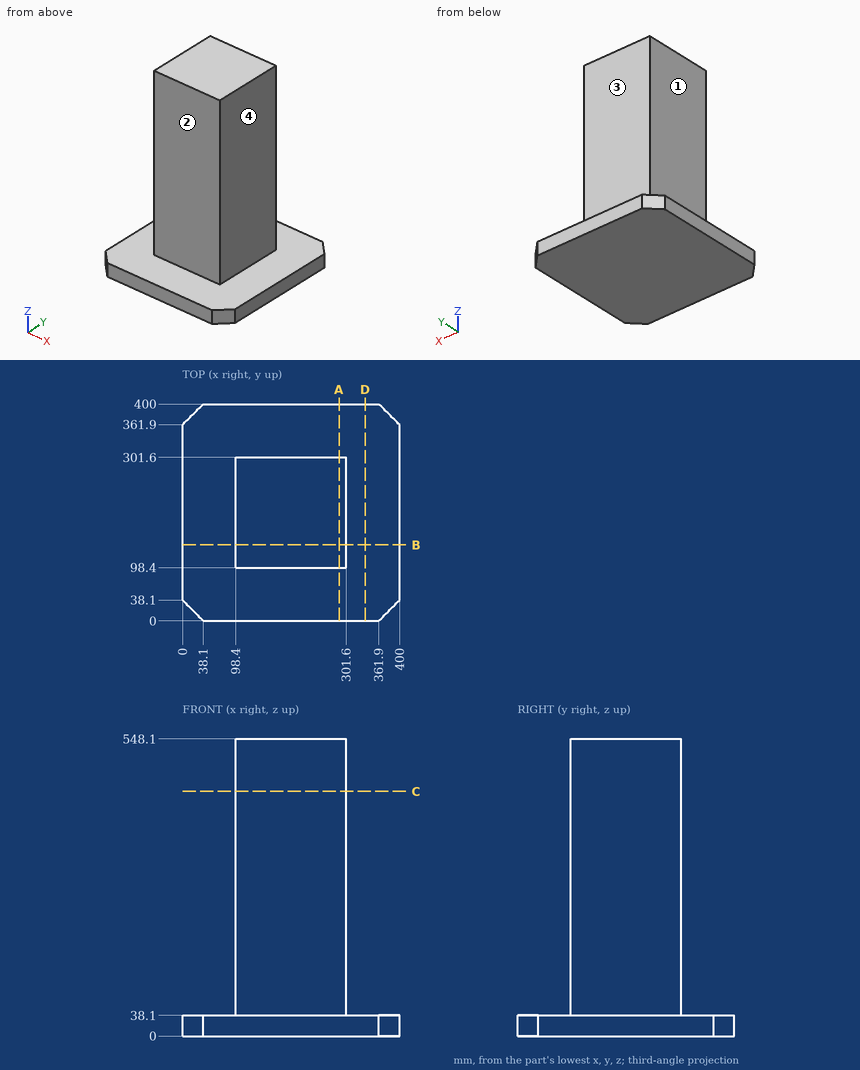
The drawing under review shows one solid part. Ordinate dimensions are in mm from its lowest x, y, z. A direction names the side the tool comes from. Give positions to 0.01 mm unless a question says otherwise; leave off trailing zeros. Write each loop counter-clockwise with the first axis right and the second up, starting at its lowest first coordinate (ties: lowest second). Pieces come first, ordered by that corner, then holes. Notation, with made-up numbers: (56, 33) -> (81, 33) arc R21 ccw to (81, 61) -> close; hole circle Ø9 at (-5.5, -10.5). An arc over 180 degrees is marked (long way). Use CSV: the item, a comma, the result in double quotes.
Q1. For P1, Ø1, axis at x = 122.5, z = 311.5, coming from the -Y side; P2, Ø1.5, axis at x = 269.5, y = 337, coming from the +Z side; P3, Ø4, axis at y = 180.5, z = 312.5, coming from the +X side, all flat-tipped, find the tip position at first contact; note any pin that passes through.
Conclusion:
P1,"y = 98.4"
P2,"z = 38.1"
P3,"x = 301.6"
Q2. Take a section at D-D, the plane x = 336.5. Write out the cut boundary in (y, z).
Conclusion:
outline,"(0, 0) -> (400, 0) -> (400, 38.1) -> (0, 38.1) -> close"
Q3. Take a section at C-C, the plane z = 451. Write out the cut boundary in (x, y).
Conclusion:
outline,"(98.4, 98.4) -> (301.6, 98.4) -> (301.6, 301.6) -> (98.4, 301.6) -> close"
Q4. To check wall thickness, follow probe 1 along X at (y, z) = (203.5, 42); probe 2 along Z at (x, y) = (313.5, 200.5). State the ranges of each line that lie inside material, in increasing order. Write a range as [from, to].
Conclusion:
probe 1,"[98.4, 301.6]"
probe 2,"[0, 38.1]"
Q5. Tool access review of the marked faces 1, 2, 3 and 4: name each direction out of +Z, -Z, +X, -X, +Y, -Y from which nothing blocks a thin tool from reaching the whole face with its end or side.
Conclusion:
face 1,"+Z, -X, +Y, -Y"
face 2,"+Z, +X, -X, -Y"
face 3,"+Z, +X, -X, +Y"
face 4,"+Z, +X, +Y, -Y"
Q6. Take a section at A-A, the plane x = 288.5. Write out the cut boundary in (y, z), then the cut area to 3 significant figures.
Conclusion:
outline,"(0, 0) -> (400, 0) -> (400, 38.1) -> (301.6, 38.1) -> (301.6, 548.1) -> (98.4, 548.1) -> (98.4, 38.1) -> (0, 38.1) -> close"
area,"119,000 mm2"
